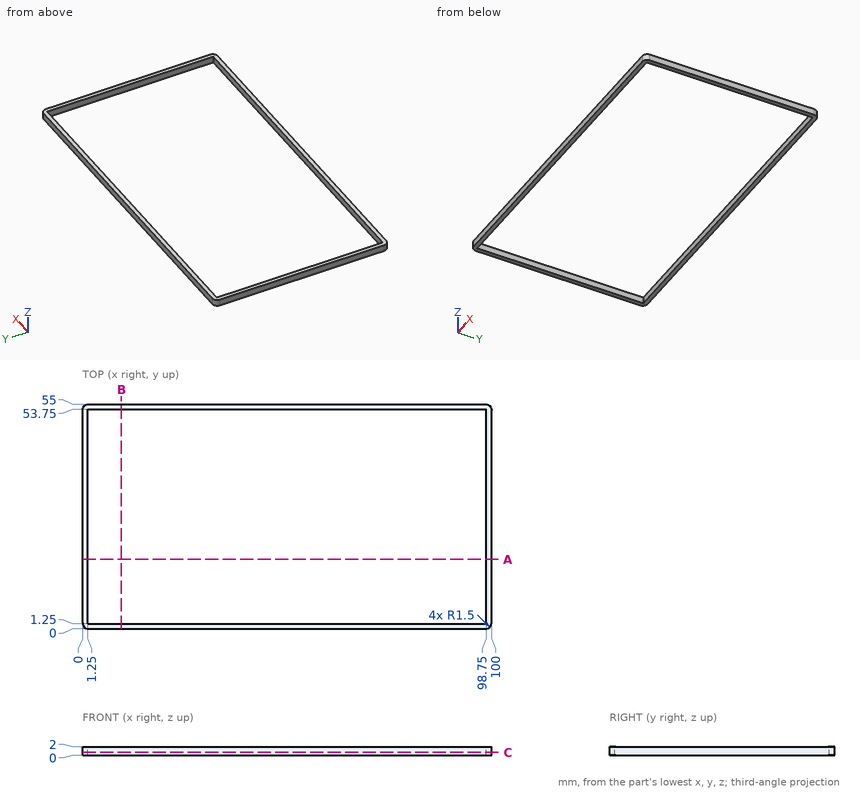
Part print with two shaded views. Sizes in mm from the minimum x, y, z corner. Round coordinates to 2 decimals unless told otherwise and drop trailing zeros. Loops run counter-clockwise (first coordinate to the right, second up) from the corner with the lowest first, then second, coordinate; pieces in that order, holes last.
Item 1: Drill centre lines: line 1 along X through (y, z) = (29, 0.6); line 2 along Y through (x, z) = (95, 0.75). Where is each one in solid material? Low to high.
Item 2: Saw through at B-B (x = 9.5). List the corners of the cut face in (y, z).
Item 3: Saw through at C-C (z = 0.7). List the corners of the cut face in (x, y), then the cut area to 3 significant figures.
Item 4: Saw through at A-A (y = 17). List the corners of the cut face in (x, z), then the cut area to 3 significant figures.
Worked answers:
1. line 1: x = 0 to 1.25, 98.75 to 100
1. line 2: y = 0 to 1.25, 53.75 to 55
2. outline: (0, 0) - (1.25, 0) - (1.25, 2) - (0, 2) - close; (53.75, 0) - (55, 0) - (55, 2) - (53.75, 2) - close
3. outline: (0, 1.5) arc R1.5 ccw to (1.5, 0) - (98.5, 0) arc R1.5 ccw to (100, 1.5) - (100, 53.5) arc R1.5 ccw to (98.5, 55) - (1.5, 55) arc R1.5 ccw to (0, 53.5) - close; hole (1.25, 1.25) - (98.75, 1.25) - (98.75, 53.75) - (1.25, 53.75) - close
3. area: 379 mm2
4. outline: (0, 0) - (1.25, 0) - (1.25, 2) - (0, 2) - close; (98.75, 0) - (100, 0) - (100, 2) - (98.75, 2) - close
4. area: 5.00 mm2
